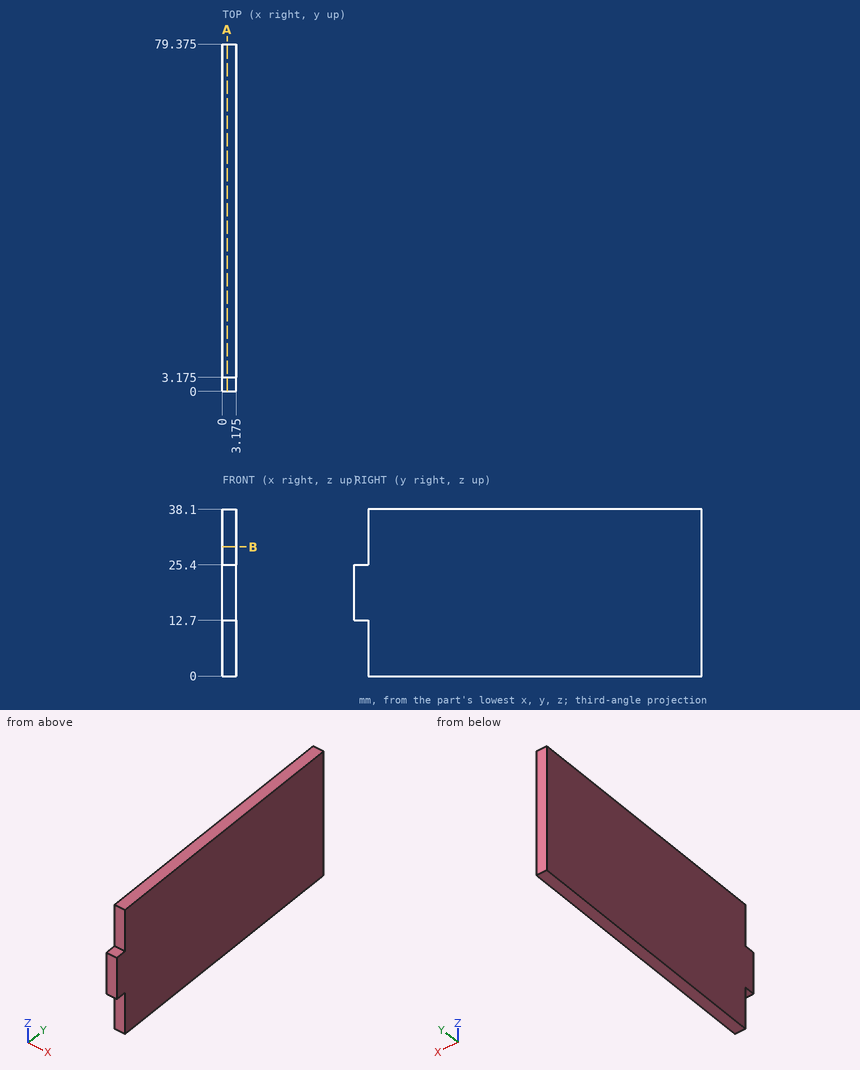
Source: three-view drawing plus pictorial views. Frame: mm from the lowest corner of the part. Give positions to 0.01 mm unless a question says otherwise; leave off trailing zeros. Write each loop counter-clockwise with the first axis right and the second up, starting at its lowest first coordinate (ties: lowest second). Pieces come first, ordered by that corner, then holes. Notation, with made-up numbers: M 82.5,17.5 L 87.5,17.5 A10 cw 87.5,25.5 Z; hole C -5.75,59 d3. An arc over 180 degrees is marked long. Use one line per item in the form item = value.
1. Cut plane B-B on z = 29.5. Return loops of the section in (x, y) (3 decimals), and give its area (3 significant figures).
Outcome:
outline = M 0,3.175 L 3.175,3.175 L 3.175,79.375 L 0,79.375 Z
area = 242 mm²
2. First-contact query: P1, Ø1, axis at x = 1.5, y = 1, coming from the +Z side; P2, Ø1, axis at x = 2, y = 2, coming from the -Z side. Flat tips, straight axial feed; report the tip coordinate or a pass-through.
Outcome:
P1 = 25.4
P2 = 12.7
3. Ray query, L1, parallel to Y at x = 2.6, z = 33 (3 decimals). Return the intervals inside material, ascending.
Outcome:
L1 = 3.175 to 79.375
4. Cut plane A-A on x = 1.1. Return loops of the section in (y, z) (3 decimals), and give its area (3 significant figures).
Outcome:
outline = M 0,12.7 L 3.175,12.7 L 3.175,0 L 79.375,0 L 79.375,38.1 L 3.175,38.1 L 3.175,25.4 L 0,25.4 Z
area = 2,940 mm²
